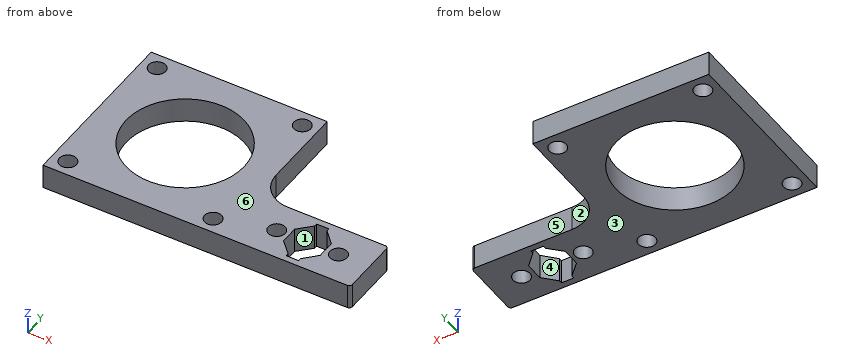
from build123d import *

# Parameters (mm, degrees)
STEPPER_PLATE_SKETCH_R   = 19.1
PLATE_BOSS_EXTRUDE_DEPTH = 8
FILLET1_R                = 10
FILLET2_R                = 1
M5_CLEARANCE_HOLE1_D     = 5.5


with BuildPart() as part:
    # Stepper Plate Sketch → Plate Boss-Extrude (new body)
    with BuildSketch(Plane.XY):
        Polygon((-22.536751464, 8), (-79.536751464, 8), (-79.536751464, -49), (20, -49), (20, -29), (-22.536751464, -29), align=None)
        with Locations((-51.036751464, -20.5)):
            Circle(STEPPER_PLATE_SKETCH_R, mode=Mode.SUBTRACT)
        Polygon((-2, -31), (2, -31), (2, -32), (5.88, -36.06), (5.88, -41.94), (2, -46), (2, -47), (-2, -47), (-2, -46), (-6, -41.94), (-6, -36.06), (-2, -32), align=None, mode=Mode.SUBTRACT)
    extrude(amount=-PLATE_BOSS_EXTRUDE_DEPTH)

    # Fillet1
    fillet1_edges = [part.edges().sort_by_distance(p)[0] for p in [
        (-22.536751464, -29, -4),
    ]]
    fillet(fillet1_edges, radius=FILLET1_R)

    # Fillet2
    fillet2_edges = [part.edges().sort_by_distance(p)[0] for p in [
        (20, -29, -4),
        (20, -49, -4),
    ]]
    fillet(fillet2_edges, radius=FILLET2_R)

    # M5 Clearance Hole1 (through all)
    with Locations(Plane.XY):
        with Locations((-74.536751464, 3), (-74.536751464, -44), (-27.536751464, -44), (-27.536751464, 3), (-10, -39), (10, -39)):
            Hole(M5_CLEARANCE_HOLE1_D / 2)


solid = part.part
Geometry check sheet. Reference: the model listing, model coordinates, mm. Face numbers are marked on the shaded views. A direction names the side the tool comes from. Give positions to 0.01 mm unless a question says otherwise; leave off trailing zeros. Write each loop counter-clockwise with the first axis right and the second up, starting at its lowest first coordinate (ties: lowest second). Pieces come first, ordered by that corner, then holes. Notation, with made-up numbers: M -7,83 L 20,83 A10 ccw 20,99 Z; hole C 8,-36 d7. An arc over 180 degrees is marked long. Answer as CSV lines item,"result". Start each with the question number.
Q1. Go/stop test with flat-tipped pins: pin 1 (4 mm diameter, centred on y = -2, z = -5.5, fed in from +X); pin 2 (3 mm diameter, centred on x = -1, z = -4.5, fed in from +Y); pin 3 (5 mm diameter, centred on x = -74.54, y = -44, fed in from -Z). Record where each tip stops, or that it passes through.
Q2. Material ranges on L1, parallel to Y at x = -73.5, z = -2.75; L2, parallel to Y at x = 10, z = -4; L3, parallel to X at y = -25, z = -4.5, recorded low to high.
Q3. Section check B-B, the plane x = -10. Record the cut outline in (y, z), then the cut area to 3 significant figures.
Q4. Section check D-D, the plane z = -5.75. Give the number of separate pieces and of enclosed holes in the cut face, then the cut area to 3 significant figures.
Q5. Tool access check on the marked faces 4, 5 and 6. Record the directions out of +Z, -Z, +X, -X, +Y, -Y that give a thin tool (end or side, any length) a straight path to the whole face; none if there is none.
Q6. Section check A-A, the plane y = 3. Record the cut outline in (x, z).
Q7. Section check C-C, the plane y = -44. Record the cut outline in (x, z).
Q8. Release check for a two-part mould opening along X. For the marked faces 1, 2 and 3 record: pulls with the +X half, pulls with the -X half, needs draft (parallel to the pull), parting line crosses it, or undercut.
Geometry says:
1,pin 1,"x = -22.54"
1,pin 2,"y = -29"
1,pin 3,"through"
2,L1,"-49 to -46.55, -41.45 to 0.45, 5.55 to 8"
2,L2,"-49 to -41.75, -36.25 to -29"
2,L3,"-79.54 to -69.6, -32.47 to -20.54"
3,outline,"M -49,-8 L -41.75,-8 L -41.75,0 L -49,0 Z; M -36.25,-8 L -29,-8 L -29,0 L -36.25,0 Z"
3,area,"116 mm^2"
4,separate pieces,"1"
4,enclosed holes,"8"
4,area,"2,690 mm^2"
5,face 4,"+Z, -Z"
5,face 5,"+Z, -Z, +X, +Y"
5,face 6,"+Z, +X, -X, +Y, -Y"
6,outline,"M -79.54,-8 L -77.29,-8 L -77.29,0 L -79.54,0 Z; M -71.79,-8 L -30.29,-8 L -30.29,0 L -71.79,0 Z; M -24.79,-8 L -22.54,-8 L -22.54,0 L -24.79,0 Z"
7,outline,"M -79.54,-8 L -77.29,-8 L -77.29,0 L -79.54,0 Z; M -71.79,-8 L -30.29,-8 L -30.29,0 L -71.79,0 Z; M -24.79,-8 L -3.97,-8 L -3.97,0 L -24.79,0 Z; M 3.91,-8 L 20,-8 L 20,0 L 3.91,0 Z"
8,face 1,"undercut"
8,face 2,"pulls with the +X half"
8,face 3,"needs draft"
